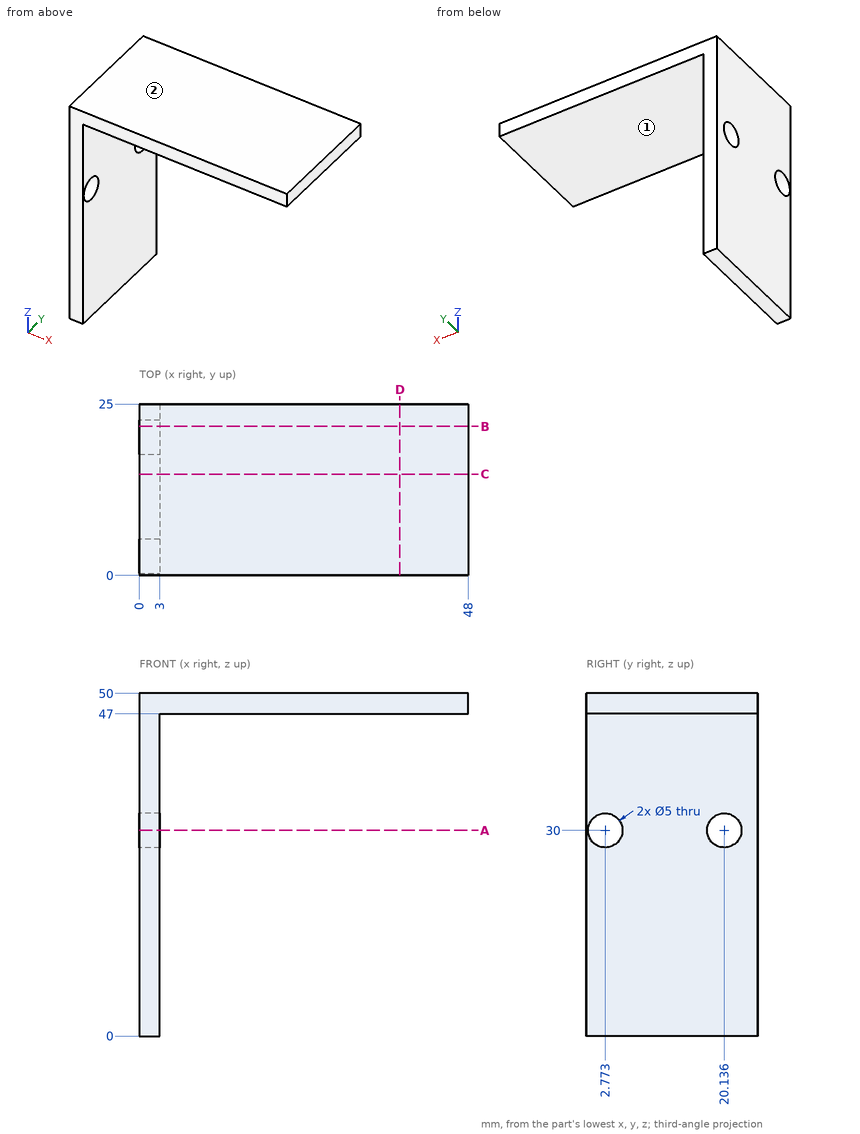
Can you work these out from the drawing? Everything is in mm from the part's minimum corner. A direction names the side the tool comes from. Coordinates: 2 decimals unless noted, no trailing zeros. Order: outer loops, then holes, each group sorted by start corner. A loop starts at its lowest first (then second) coordinate and runs counter-clockwise, first axis right, second up. Notation, with made-up numbers: (-2, 69.5) -> (57, 69.5) arc R10 ccw to (57, 88.5) -> close; hole circle Ø1 at (42, -16.5). An arc over 180 degrees is marked (long way). Return JSON: item names as keys, results as strings.
1) If we section it at A-A on z = 30: State how many separate pieces and enclosed holes the cut face has, plus the area to 3 significant figures.
Conclusion:
{"separate pieces": "3", "enclosed holes": "0", "area": "45.0 mm²"}
2) If we section it at C-C on y = 14.75: List the corners of the cut face in (x, z) for me, plus the area to 3 significant figures.
Conclusion:
{"outline": "(0, 0) -> (3, 0) -> (3, 47) -> (48, 47) -> (48, 50) -> (0, 50) -> close", "area": "285 mm²"}
3) If we section it at B-B on y = 21.75: List the corners of the cut face in (x, z) for me.
Conclusion:
{"outline": "(0, 0) -> (3, 0) -> (3, 28.09) -> (0, 28.09) -> close; (0, 31.91) -> (3, 31.91) -> (3, 47) -> (48, 47) -> (48, 50) -> (0, 50) -> close"}
4) If we section it at D-D on x = 38: List the corners of the cut face in (y, z) for me, plus the area to 3 significant figures.
Conclusion:
{"outline": "(0, 47) -> (25, 47) -> (25, 50) -> (0, 50) -> close", "area": "75.0 mm²"}
5) On a 3-axis mill with a long thin cutter (end or side, diameter ignored), from which of +Z, -Z, +X, -X, +Y, -Y can I reach the whole of each face in a straight line? I mean the marked faces 1 and 2. Say none if no direction works.
Conclusion:
{"face 1": "-Z, +X, +Y, -Y", "face 2": "+Z, +X, -X, +Y, -Y"}
6) If I drill on probe 1 along Z at (x, y) = (32, 11.25); probe 2 along X at (y, z) = (13, 6.5), over which ranges is the centre line in solid material (lowest first)?
Conclusion:
{"probe 1": "z = 47 to 50", "probe 2": "x = 0 to 3"}
7) I'm going to push flat-ended pins straight in: P1, Ø4, axis at x = 11, y = 3.5, coming from the -Z side; P2, Ø5, axis at y = 12, z = 15, coming from the +X side. Where does each tip first touch, or does it pass through?
Conclusion:
{"P1": "stops at z = 47", "P2": "stops at x = 3"}
